from build123d import *

# Parameters (mm, degrees)
F1_DEPTH     = 30
F2_T         = -2.5
F4_DEPTH     = 2.5
F5_T1_DEPTH  = 83
F5_T3_DEPTH  = 41
F5_T6_ANGLE  = 90
F5_T8_ANGLE  = 90
F5_T10_ANGLE = 90
F5_T12_ANGLE = 90


# Not quite as in the source:
# - a fillet or chamfer that OpenCascade refuses, or shapes differently, is made with other operations: its cross-section is extruded or revolved along the edge and cut away or added


with BuildPart() as f1:
    # F0 (on Top) → F1 (new body)
    with BuildSketch(Plane.XY):
        with BuildLine():
            ThreePointArc((32.5, 41.5), (28.9852813742, 49.9852813742), (20.5, 53.5))
            Line((20.5, 53.5), (-20.5, 53.5))
            ThreePointArc((-20.5, 53.5), (-28.9852813742, 49.9852813742), (-32.5, 41.5))
            Line((-32.5, 41.5), (-32.5, -41.5))
            ThreePointArc((-32.5, -41.5), (-28.9852813742, -49.9852813742), (-20.5, -53.5))
            Line((-20.5, -53.5), (20.5, -53.5))
            ThreePointArc((20.5, -53.5), (28.9852813742, -49.9852813742), (32.5, -41.5))
            Line((32.5, -41.5), (32.5, 41.5))
        make_face()
    extrude(amount=F1_DEPTH)

    # F2
    f2_openings = [f1.faces().sort_by_distance(p)[0] for p in [
        (0, 0, 30),
    ]]
    offset(amount=F2_T, openings=f2_openings)

    # F3 (on face) → F4 (join)
    with BuildSketch(Plane.XY.offset(30)):
        with BuildLine():
            Line((-20.5, -58.5), (20.5, -58.5))
            ThreePointArc((20.5, -58.5), (32.5208152802, -53.5208152802), (37.5, -41.5))
            Line((37.5, -41.5), (37.5, 41.5))
            ThreePointArc((37.5, 41.5), (32.5208152802, 53.5208152802), (20.5, 58.5))
            Line((20.5, 58.5), (-20.5, 58.5))
            ThreePointArc((-20.5, 58.5), (-32.5208152802, 53.5208152802), (-37.5, 41.5))
            Line((-37.5, 41.5), (-37.5, -41.5))
            ThreePointArc((-37.5, -41.5), (-32.5208152802, -53.5208152802), (-20.5, -58.5))
        make_face()
        with BuildLine():
            ThreePointArc((20.5, 53.5), (28.9852813742, 49.9852813742), (32.5, 41.5))
            Line((32.5, 41.5), (32.5, -41.5))
            ThreePointArc((32.5, -41.5), (28.9852813742, -49.9852813742), (20.5, -53.5))
            Line((20.5, -53.5), (-20.5, -53.5))
            ThreePointArc((-20.5, -53.5), (-28.9852813742, -49.9852813742), (-32.5, -41.5))
            Line((-32.5, -41.5), (-32.5, 41.5))
            ThreePointArc((-32.5, 41.5), (-28.9852813742, 49.9852813742), (-20.5, 53.5))
            Line((-20.5, 53.5), (20.5, 53.5))
        make_face(mode=Mode.SUBTRACT)
        with BuildLine():
            Line((32.5, -41.5), (32.5, 41.5))
            ThreePointArc((32.5, 41.5), (28.9852813742, 49.9852813742), (20.5, 53.5))
            Line((20.5, 53.5), (-20.5, 53.5))
            ThreePointArc((-20.5, 53.5), (-28.9852813742, 49.9852813742), (-32.5, 41.5))
            Line((-32.5, 41.5), (-32.5, -41.5))
            ThreePointArc((-32.5, -41.5), (-28.9852813742, -49.9852813742), (-20.5, -53.5))
            Line((-20.5, -53.5), (20.5, -53.5))
            ThreePointArc((20.5, -53.5), (28.9852813742, -49.9852813742), (32.5, -41.5))
        make_face()
        with BuildLine():
            Line((-20.5, 51), (20.5, 51))
            ThreePointArc((20.5, 51), (27.2175144213, 48.2175144213), (30, 41.5))
            Line((30, 41.5), (30, -41.5))
            ThreePointArc((30, -41.5), (27.2175144213, -48.2175144213), (20.5, -51))
            Line((20.5, -51), (-20.5, -51))
            ThreePointArc((-20.5, -51), (-27.2175144213, -48.2175144213), (-30, -41.5))
            Line((-30, -41.5), (-30, 41.5))
            ThreePointArc((-30, 41.5), (-27.2175144213, 48.2175144213), (-20.5, 51))
        make_face(mode=Mode.SUBTRACT)
    extrude(amount=F4_DEPTH)

    # F5: fillet of radius 5 on 1 edges, made by hand

    # F5_s2 → F5_t1 (cut)
    with BuildSketch(Plane.XZ.offset(-41.5)):
        with BuildLine():
            ThreePointArc((33.1698729811, 32.5), (35.6698729811, 31.8301270189), (37.5, 30))
            Line((37.5, 30), (37.5, 32.5))
            Line((37.5, 32.5), (33.1698729811, 32.5))
        make_face()
        with BuildLine():
            ThreePointArc((-33.1698729811, 32.5), (-35.6698729811, 31.8301270189), (-37.5, 30))
            Line((-37.5, 30), (-37.5, 32.5))
            Line((-37.5, 32.5), (-33.1698729811, 32.5))
        make_face()
    extrude(amount=F5_T1_DEPTH, mode=Mode.SUBTRACT)

    # F5_s4 → F5_t3 (cut)
    with BuildSketch(Plane.YZ.offset(-20.5)):
        with BuildLine():
            ThreePointArc((58.5, 30), (56.6698729811, 31.8301270189), (54.1698729811, 32.5))
            Line((54.1698729811, 32.5), (58.5, 32.5))
            Line((58.5, 32.5), (58.5, 30))
        make_face()
        with BuildLine():
            ThreePointArc((-54.1698729811, 32.5), (-56.6698729811, 31.8301270189), (-58.5, 30))
            Line((-58.5, 30), (-58.5, 32.5))
            Line((-58.5, 32.5), (-54.1698729811, 32.5))
        make_face()
    extrude(amount=F5_T3_DEPTH, mode=Mode.SUBTRACT)

    # F5_s5 → F5_t6 (revolve, cut)
    with BuildSketch(Plane.YZ.offset(20.5)):
        with BuildLine():
            ThreePointArc((-54.1698729811, 32.5), (-56.6698729811, 31.8301270189), (-58.5, 30))
            Line((-58.5, 30), (-58.5, 32.5))
            Line((-58.5, 32.5), (-54.1698729811, 32.5))
        make_face()
    revolve(axis=Axis((20.5, -41.5, 32.5), (0, 0, 1)), revolution_arc=F5_T6_ANGLE, mode=Mode.SUBTRACT)

    # F5_s7 → F5_t8 (revolve, cut)
    with BuildSketch(Plane.XZ.offset(-41.5)):
        with BuildLine():
            ThreePointArc((33.1698729811, 32.5), (35.6698729811, 31.8301270189), (37.5, 30))
            Line((37.5, 30), (37.5, 32.5))
            Line((37.5, 32.5), (33.1698729811, 32.5))
        make_face()
    revolve(axis=Axis((20.5, 41.5, 32.5), (0, 0, 1)), revolution_arc=F5_T8_ANGLE, mode=Mode.SUBTRACT)

    # F5_s9 → F5_t10 (revolve, cut)
    with BuildSketch(Plane.YZ.offset(-20.5)):
        with BuildLine():
            ThreePointArc((54.1698729811, 32.5), (56.6698729811, 31.8301270189), (58.5, 30))
            Line((58.5, 30), (58.5, 32.5))
            Line((58.5, 32.5), (54.1698729811, 32.5))
        make_face()
    revolve(axis=Axis((-20.5, 41.5, 32.5), (0, 0, 1)), revolution_arc=F5_T10_ANGLE, mode=Mode.SUBTRACT)

    # F5_s11 → F5_t12 (revolve, cut)
    with BuildSketch(Plane.XZ.offset(41.5)):
        with BuildLine():
            ThreePointArc((-33.1698729811, 32.5), (-35.6698729811, 31.8301270189), (-37.5, 30))
            Line((-37.5, 30), (-37.5, 32.5))
            Line((-37.5, 32.5), (-33.1698729811, 32.5))
        make_face()
    revolve(axis=Axis((-20.5, -41.5, 32.5), (0, 0, 1)), revolution_arc=F5_T12_ANGLE, mode=Mode.SUBTRACT)


solid = f1.part
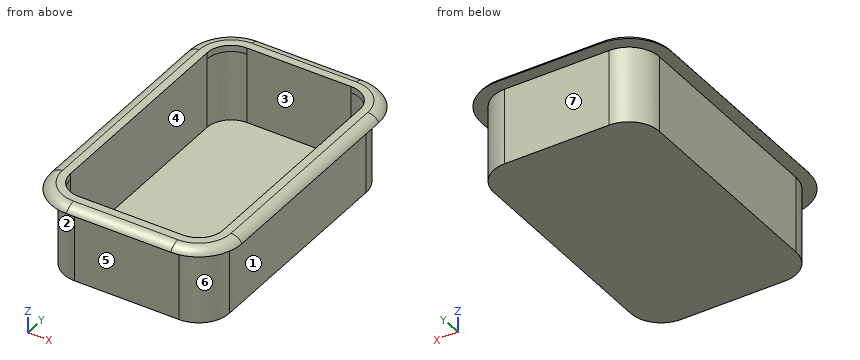
Work out the finished part from the listing and answer in its coordinate system (mm). Face numbers are marked on the shaded views. A direction names the side the tool comes from. Round coordinates to 2 decimals unless told otherwise and drop trailing zeros. Order: outer loops, then holes, each group sorted by start corner. A loop starts at its lowest first (then second) coordinate and runs counter-clockwise, first axis right, second up. Notation, with made-up numbers: M 13,82 L 63,82 A12 cw 63,88 Z; hole C 46.5,35 d8. An arc over 180 degrees is marked long. Put each result on its own line as item: value. Start each with the question number.
Q1. For a pull along Y with two mould halves and no side action, classify the marked faces 1, 2, 3 and 4 as pulls with the +Y half, pulls with the -Y half, needs draft (parallel to the pull), parting line crosses it, or undercut.
Q2. Section C-C, the plane x = -13 is taken. Write down the section's boundary in (y, z), and give its area (3 significant figures).
Q3. A tool of negligible diameter and unlimited length cuts with its end or side. For the marked faces 5, 6 and 7, from which of +Z, -Z, +X, -X, +Y, -Y can it reach the whole face along a straight path? Write none if from no direction.
Q4. Section B-B, the plane y = 24 is taken. Write down the section's boundary in (x, z).
Q5. Flat-ended cylindrical pins translate along their axes: pin 1 (15 mm diameter, centred on x = -10, z = 24.5, fed in from +Y); pin 2 (8 mm diameter, centred on x = -24, y = 25, fed in from -Z); pin 3 (15 mm diameter, centred on y = -3.5, z = 17.5, fed in from -X); pin 4 (12 mm diameter, centred on x = 14.5, y = 16, fed in from +Z). Find the tip coordinate at first contact, or state that the pin passes through.
Q6. Straight lines are drawn through the part: L1, parallel to Y at x = -18, z = 11; L2, parallel to X at y = 1, z = 4; L3, parallel to Z at x = 21.5, y = -3. For each, find the intervals that lie inside material, in ascending order. Write a range as [from, to].
Q7. Section A-A, the plane z = 23.5 is taken. Write down the section's boundary in (x, y), and give its area (3 significant figures).
Findings below:
1. face 1: needs draft
1. face 2: pulls with the -Y half
1. face 3: undercut
1. face 4: undercut
2. outline: M -58.5,30 L -53.5,30 L -53.5,0 L 53.5,0 L 53.5,30 L 58.5,30 A5 ccw 54.17,32.5 L 51,32.5 L 51,2.5 L -51,2.5 L -51,32.5 L -54.17,32.5 A5 ccw Z
2. area: 436 mm^2
3. face 5: -Z, +X, -X, -Y
3. face 6: -Z, +X, -Y
3. face 7: -Z, +X, -X, +Y
4. outline: M -37.5,30 L -32.5,30 L -32.5,0 L 32.5,0 L 32.5,30 L 37.5,30 A5 ccw 33.17,32.5 L 30,32.5 L 30,2.5 L -30,2.5 L -30,32.5 L -33.17,32.5 A5 ccw Z
5. pin 1: stops at y = 58.5
5. pin 2: stops at z = 0
5. pin 3: stops at x = -32.5
5. pin 4: stops at z = 2.5
6. L1: y = [-53.5, -51], [51, 53.5]
6. L2: x = [-32.5, -30], [30, 32.5]
6. L3: z = [0, 2.5]
7. outline: M -32.5,-41.5 A12 ccw -20.5,-53.5 L 20.5,-53.5 A12 ccw 32.5,-41.5 L 32.5,41.5 A12 ccw 20.5,53.5 L -20.5,53.5 A12 ccw -32.5,41.5 Z; hole M -30,-41.5 A9.5 ccw -20.5,-51 L 20.5,-51 A9.5 ccw 30,-41.5 L 30,41.5 A9.5 ccw 20.5,51 L -20.5,51 A9.5 ccw -30,41.5 Z
7. area: 789 mm^2
